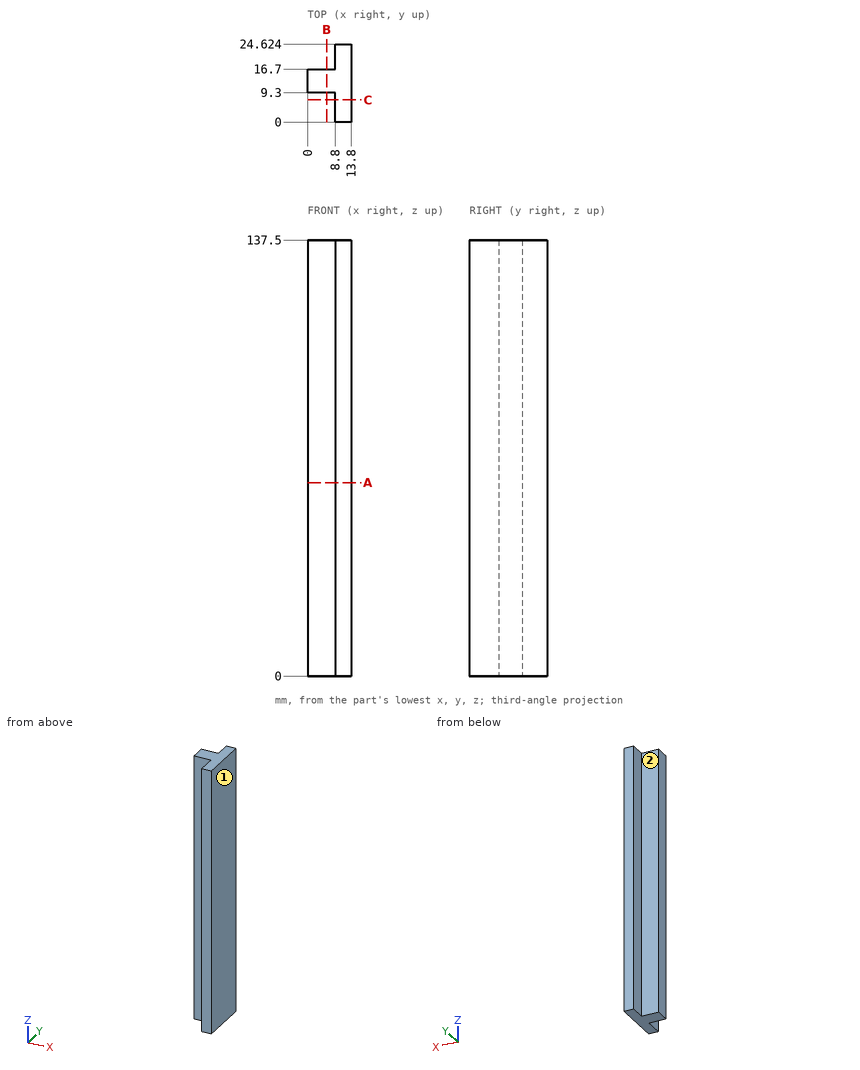
The figure shows three views and two pictorial views of one solid part (mm, origin at its lowest corner). Answer the questions. A direction names the side the tool comes from. Give positions to 0.01 mm unless a question says otherwise; leave off trailing zeros. Order: outer loops, then holes, each group sorted by start corner. A loop starts at its lowest first (then second) coordinate and runs counter-clockwise, first axis right, second up. Notation, with made-up numbers: (50.25, 67) -> (106.25, 67) arc R32 ccw to (106.25, 95) -> close; hole circle Ø10 at (20, 0.5). An arc over 180 degrees is marked (long way). One line per item, written item: value.
1) Find section A-A, the plane z = 61. Determine the outline of the cut face in (x, y).
Reported:
outline: (0, 9.3) -> (8.8, 9.3) -> (8.8, 0) -> (13.8, 0) -> (13.8, 24.62) -> (8.8, 24.62) -> (8.8, 16.7) -> (0, 16.7) -> close
2) Find section B-B, the plane x = 6. Determine the outline of the cut face in (y, z), plus the area to 3 significant figures.
Reported:
outline: (9.3, 0) -> (16.7, 0) -> (16.7, 137.5) -> (9.3, 137.5) -> close
area: 1,020 mm^2
3) A tool of negligible diameter and unlimited length cuts with its end or side. For the marked faces 1 and 2, from which of +Z, -Z, +X, -X, +Y, -Y can it reach the whole face along a straight path? Write none if from no direction.
Reported:
face 1: +Z, -Z, +X, +Y, -Y
face 2: +Z, -Z, -X, +Y
4) Find section C-C, the plane y = 7. Determine the outline of the cut face in (x, z).
Reported:
outline: (8.8, 0) -> (13.8, 0) -> (13.8, 137.5) -> (8.8, 137.5) -> close
5) Find the intervals of material crossed by line 1 (X direction, y = 1.75, z = 125); line 2 (Y direction, x = 4.75, z = 23.5), in increasing order.
Reported:
line 1: x = 8.8 to 13.8
line 2: y = 9.3 to 16.7
6) Flat-ended cylindrical pins translate along their axes: P1, Ø4, axis at y = 21.5, z = 84.5, coming from the -X side; P2, Ø6, axis at x = 3, z = 40, coming from the +Y side; P3, Ø7, axis at x = 5, z = 85.5, coming from the -Y side. Find the tip coordinate at first contact, or state that the pin passes through.
Reported:
P1: stops at x = 8.8
P2: stops at y = 16.7
P3: stops at y = 9.3
